Could you check a few things on this drawing? It's one solid part, dimensions in mm from its lowest x, y, z. Give positions to 0.01 mm unless a question says otherwise; leave off trailing zeros. Order: outer loops, then holes, each group sorted by start corner. A loop starts at its lowest first (then second) coordinate and runs counter-clockwise, first axis right, second up. Notation, with made-up numbers: M 48,88 L 95,88 A31 ccw 95,127 Z; hole C 87.5,-16.75 d8. An arc over 180 degrees is marked long. Return JSON: item names as keys, results as strings. Group by question number.
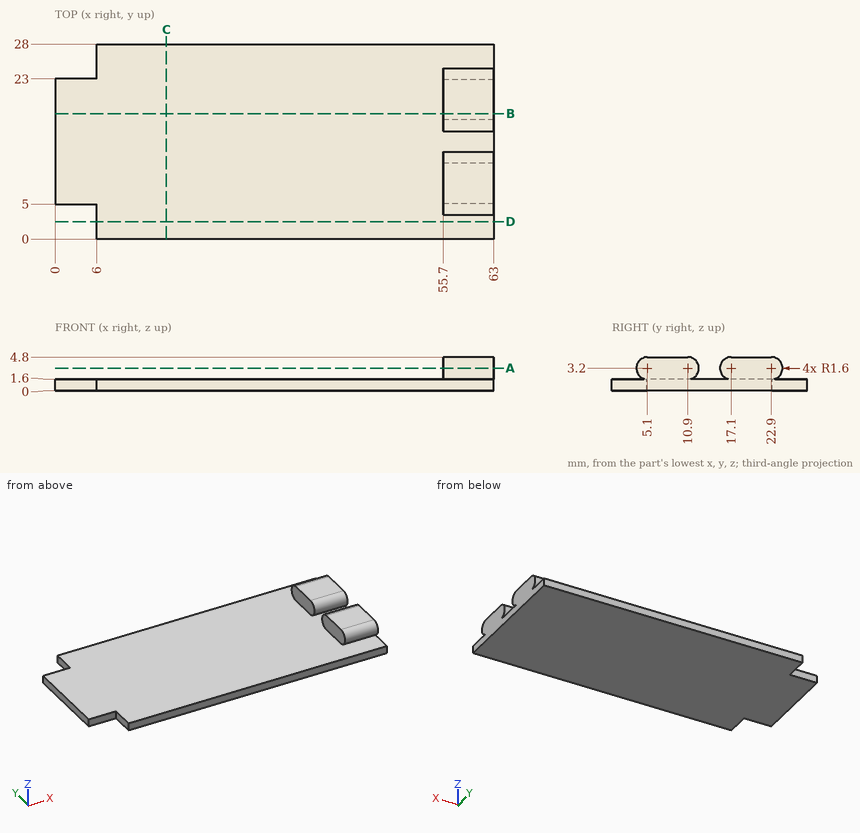
1. Imagine slicing it at A-A, the plane z = 3.2. Please give me the cut outline in (x, y).
2. For pin 1 (10 mm diameter, centred on x = 33.5, y = 5, fed in from +Z); pin 2 (1 mm diameter, centred on y = 9, z = 2.5, fed in from -X); pin 3 (0.5 mm diameter, centred on y = 3.5, z = 0.5, fed in from -X); pin 4 (1.5 mm diameter, centred on x = 44, z = 4, fed in from -Y), each with a flat end and sliding along its axis, tell me the tip position at first contact or that it passes through.
3. I need wall thicknesses on L1, parallel to X at y = 18, z = 3.25; L2, parallel to Y at x = 3, z = 0.65; L3, parallel to Z at x = 19, y = 17. Which ranges of each line are inside material? Lowest first, please. Write a range as from..to.
4. Imagine slicing it at C-C, the plane x = 16. Please give me the cut outline in (y, z).
5. Imagine slicing it at D-D, the plane y = 2.5. Please give me the cut outline in (x, z), plus the area to 3 significant figures.
6. Imagine slicing it at B-B, the plane y = 18. Please give me the cut outline in (x, z).
Values:
{
 "1": {"outline": "M 55.7,3.5 L 63,3.5 L 63,12.5 L 55.7,12.5 Z; M 55.7,15.5 L 63,15.5 L 63,24.5 L 55.7,24.5 Z"},
 "2": {"pin 1": "stops at z = 1.6", "pin 2": "stops at x = 55.7", "pin 3": "stops at x = 6", "pin 4": "passes through"},
 "3": {"L1": "x = 55.7..63", "L2": "y = 5..23", "L3": "z = 0..1.6"},
 "4": {"outline": "M 0,0 L 28,0 L 28,1.6 L 0,1.6 Z"},
 "5": {"outline": "M 6,0 L 63,0 L 63,1.6 L 6,1.6 Z", "area": "91.2 mm²"},
 "6": {"outline": "M 0,0 L 63,0 L 63,4.8 L 55.7,4.8 L 55.7,1.6 L 0,1.6 Z"}
}
